Geometry check sheet. Reference: drawing and pictorial views, mm from the part's lowest x, y, z. A direction names the side the tool comes from. Round coordinates to 2 decimals unless told otherwise and drop trailing zeros. Loops run counter-clockwise (first coordinate to the right, second up) from the corner with the lowest first, then second, coordinate; pieces in that order, holes last. Notation, with made-up numbers: (50.25, 68.25) - (102.25, 68.25) arc R22 cw to (102.25, 85.25) - close; hole circle Ø2 at (-22.5, 24.25). An arc over 180 degrees is marked (long way). Answer as CSV lines item,"result". Start each with the question number.
1) Cross-section at D-D on y = 21.59. Record the boundary of the cut face in (x, z), and give its area (3 significant figures).
2) Depth check by flat-ended pin: P1, Ø8.5, axis at x = 31.75, y = 21.59, coming from the -Z side; P2, Ø1.5, axis at x = 20.5, z = 5.5, coming from the +Y side; P3, Ø4, axis at x = 22.5, z = 15, coming from the +Y side. Enter the tip coordinate at first touch or a pass-through.
3) Cross-section at A-A on x = 31.75. State how many separate pieces and enclosed holes the cut face has, and give its area (3 significant figures).
4) Draft check along X on the marked faces 3, 4, 5 and 6. Enter one of: released by +X, released by -X, zero draft, split by the parting line, or undercut.
5) Access from +Z, -Z, +X, -X, +Y, -Y to the whole of each face (thin tool, end or side, straight path). Record for the marked faces 1 and 2.
6) Thickness scan on line 1 along X through (y, z) = (5.25, 12.7) (1 decimal); line 2 along Z through (x, y) = (38, 16); line 3 along Z through (x, y) = (13, 5). Record the ranges inside material, lowest first.
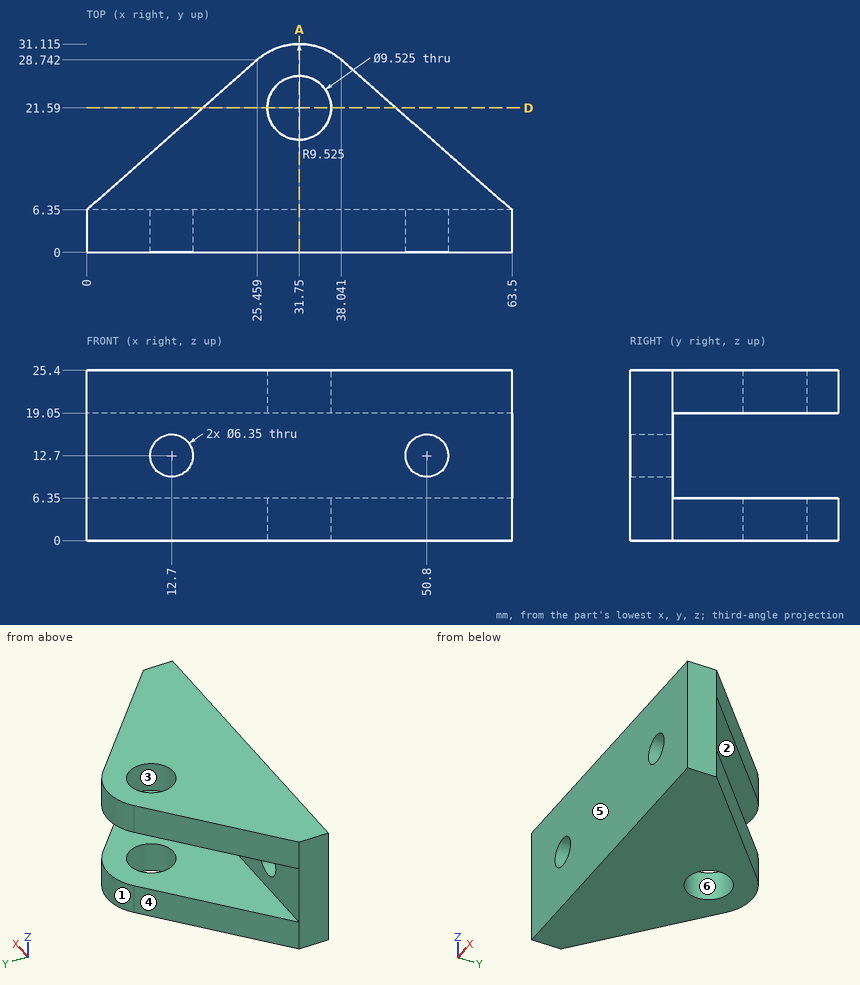
Answer block:
1,outline,"(17.33, 0) - (26.99, 0) - (26.99, 6.35) - (17.33, 6.35) - close; (17.33, 19.05) - (26.99, 19.05) - (26.99, 25.4) - (17.33, 25.4) - close; (36.51, 0) - (46.17, 0) - (46.17, 6.35) - (36.51, 6.35) - close; (36.51, 19.05) - (46.17, 19.05) - (46.17, 25.4) - (36.51, 25.4) - close"
1,area,"245 mm^2"
2,P1,"passes through"
2,P2,"stops at y = 25.04"
2,P3,"stops at y = 6.35"
3,separate pieces,"3"
3,enclosed holes,"0"
3,area,"355 mm^2"
4,face 3,"undercut"
4,face 4,"released by -X"
4,face 5,"zero draft"
4,face 6,"undercut"
5,face 1,"+Z, -Z, +Y"
5,face 2,"+X, -X, +Y"
6,line 1,"x = 0 to 9.5, 15.9 to 47.6, 54 to 63.5"
6,line 2,"z = 0 to 6.35, 19.05 to 25.4"
6,line 3,"z = 0 to 9.54, 15.86 to 25.4"
